Input: part model. Units: mm. Frame: model coordinates. Give positions to 0.01 mm unless a question says otherwise; leave off trailing zeros. Loops run counter-clockwise (first coordinate to the right, second up) from the corner with the lowest first, then second, coordinate; pieces in that order, holes last. Notation, with made-up numbers: (-9.5, 72) -> (-4.5, 72) arc R21 ccw to (-4.5, 97) -> close; hole circle Ø1 at (-15, 42.25). An arc over 180 degrees is marked (long way). One line per question, with ' | ' between items.
from build123d import *

# Parameters (mm, degrees)
F1_DEPTH = 6.35


with BuildPart() as f1:
    # F0 (on Front) → F1 (new body)
    with BuildSketch(Plane.XZ):
        Polygon((-135.90005, 38.716007), (-220.352262, 53.212889), (-220.352262, 39.346308), (-135.90005, 20.437343), (-135.90005, 25.42473), (-132.72505, 25.42473), (-132.72505, 20.241606), (-43.884959, 14.764653), (-43.884959, 19.270245), (-43.884959, 19.844653), (-40.709959, 19.844653), (-40.709959, 19.270245), (-40.709959, 14.764653), (0, 14.764653), (0, 19.844653), (3.175, 19.844653), (3.175, 14.764653), (55.669224, 14.764653), (55.669224, 19.844653), (58.844224, 19.844653), (58.844224, 14.764653), (113.651348, 20.126716), (113.651348, 25.054362), (116.826348, 25.054362), (116.826348, 20.437343), (169.136286, 33.673622), (169.136286, 45.019001), (116.826348, 38.08571), (116.826348, 33.067703), (113.651348, 33.067703), (113.651348, 37.809598), (58.844224, 33.043321), (58.844224, 27.963321), (55.669224, 27.963321), (55.669224, 33.043321), (3.175, 33.043321), (3.175, 27.963321), (0, 27.963321), (0, 33.043321), (-40.709959, 33.043321), (-40.709959, 27.963321), (-43.884959, 27.963321), (-43.884959, 33.043321), (-132.72505, 38.52027), (-132.72505, 34.656454), (-135.90005, 34.656454), align=None)
    extrude(amount=F1_DEPTH)


solid = f1.part
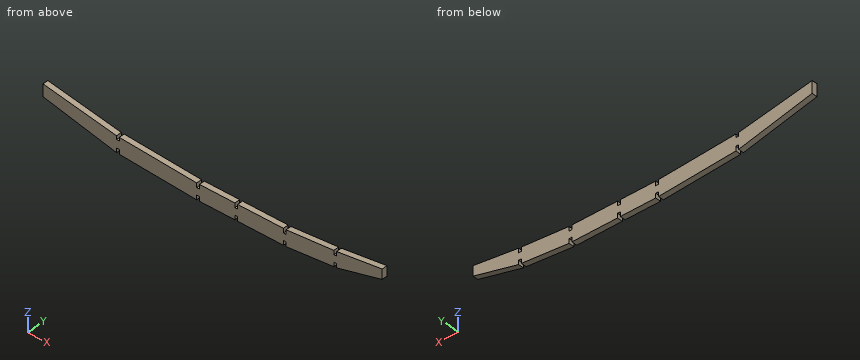
1. Ray query, line 1 along Z through (x, y) = (19.5, -4); line 2 along Z through (x, y) = (56, -4.5). Return the intervals inside material, ascending. Write a range as from..to.
Determined:
line 1: z = 14.76..33.04 | line 2: z = 19.84..27.96
2. Section query A-A (x = -147.5). Output: boundary loops of the cut face in (y, z).
Determined:
outline: (-6.35, 23.03) -> (0, 23.03) -> (0, 40.71) -> (-6.35, 40.71) -> close
3. Pin query (flat end, axial travel): P1, Ø3.5, axis at x = 116, y = -3, coming from the +Z side; P2, Ø1, axis at x = -135, y = -2.5, coming from the -Z side; P3, Ø1.6, axis at x = 2.5, y = -4.5, coming from the +Z side; P4, Ø1, axis at x = 108.5, z = 39.5, coming from the -Y side. Return the tip coordinate at first contact, or that it passes through.
Determined:
P1: stops at z = 38.21 | P2: stops at z = 25.42 | P3: stops at z = 33.04 | P4: passes through
4. Section query B-B (x = -63.5). Output: boundary loops of the cut face in (y, z).
Determined:
outline: (-6.35, 15.97) -> (0, 15.97) -> (0, 34.25) -> (-6.35, 34.25) -> close
